Autodesk Inventor part; units mm, degrees
ref_plane "YZ Plane" through (0, 0, 0) normal (1, 0, 0) x (0, 1, 0)
ref_plane "XZ Plane" through (0, 0, 0) normal (0, 1, 0) x (-1, 0, 0)
ref_plane "XY Plane" through (0, 0, 0) normal (0, 0, 1) x (1, 0, 0)
sketch "Sketch1" plane through (0, 0, 0) normal (0, 1, 0) x (-1, 0, 0)
  line L0 (25, -25) -> (-25, -25)
  line L1 (-25, -25) -> (-25, 25)
  line L2 (-25, 25) -> (25, 25)
  line L3 (25, 25) -> (25, -25)
  line L4 (25, -25) -> (-25, 25) construction
  line L5 (-25, -25) -> (25, 25) construction
  point P0 (0, 0)
  dimension "d0" = 50
  dimension "d1" = 50
extrude "Extrusion1" add sketch "Sketch1" along normal blind 10
sketch "Sketch7" plane through (0, 0, 0) normal (0, -1, 0) x (1, 0, 0)
  circle A0 centre (0, 0) radius 11.1
  line L0 (-15.5, -15.5) -> (15.5, -15.5)
  line L1 (15.5, -15.5) -> (15.5, 15.5)
  line L2 (15.5, 15.5) -> (-15.5, 15.5)
  line L3 (-15.5, 15.5) -> (-15.5, -15.5)
  line L4 (-15.5, -15.5) -> (15.5, 15.5) construction
  line L5 (15.5, -15.5) -> (-15.5, 15.5) construction
  circle A1 centre (-15.5, 15.5) radius 1.65
  circle A2 centre (-15.5, -15.5) radius 1.65
  circle A3 centre (15.5, -15.5) radius 1.65
  circle A4 centre (15.5, 15.5) radius 1.65
  dimension "d60" = 22.2
  dimension "d61" = 31
  dimension "d62" = 31
  dimension "d63" = 3.3
  dimension "d66" = 360
extrude "Extrusion6" cut sketch "Sketch7" against normal up to next contours A0 | L3 A2 L0 | L0 A2 L3 | A3 L1 L0 | L0 L1 A3 | A1 L2 L3 | L3 L2 A1 | A4 L2 L1 | L1 L2 A4
sketch "Sketch4" plane through (0, 0, 0) normal (0, -1, 0) x (1, 0, 0)
  line L0 (25, -25) -> (25, 25)
  line L1 (0, -22.2) -> (0, 22.2) construction
  line L2 (11.5, -22.2) -> (11.5, 22.2)
  line L3 (-11.5, 22.2) -> (-11.5, -22.2)
  arc A0 (-11.5, -22.2) -> (11.5, -22.2) centre (0, -22.2) ccw
  arc A1 (11.5, 22.2) -> (-11.5, 22.2) centre (0, 22.2) ccw
  line L4 (15.5, -15.5) -> (-15.5, -15.5)
  line L5 (-15.5, -15.5) -> (-15.5, 15.5)
  line L6 (-15.5, 15.5) -> (15.5, 15.5)
  line L7 (15.5, 15.5) -> (15.5, -15.5)
  line L8 (15.5, -15.5) -> (-15.5, 15.5) construction
  line L9 (-15.5, -15.5) -> (15.5, 15.5) construction
  line L10 (-15.5, -6.7) -> (-15.5, 37.7) construction
  line L11 (-13.85, -6.7) -> (-13.85, 37.7)
  line L12 (-17.15, 37.7) -> (-17.15, -6.7)
  arc A2 (-17.15, -6.7) -> (-13.85, -6.7) centre (-15.5, -6.7) ccw
  arc A3 (-13.85, 37.7) -> (-17.15, 37.7) centre (-15.5, 37.7) ccw
  line L13 (15.5, -6.7) -> (15.5, 37.7) construction
  line L14 (17.15, -6.7) -> (17.15, 37.7)
  line L15 (13.85, 37.7) -> (13.85, -6.7)
  arc A4 (13.85, -6.7) -> (17.15, -6.7) centre (15.5, -6.7) ccw
  arc A5 (17.15, 37.7) -> (13.85, 37.7) centre (15.5, 37.7) ccw
  line L16 (-15.5, -37.7) -> (-15.5, 6.7) construction
  line L17 (-13.85, -37.7) -> (-13.85, 6.7)
  line L18 (-17.15, 6.7) -> (-17.15, -37.7)
  arc A6 (-17.15, -37.7) -> (-13.85, -37.7) centre (-15.5, -37.7) ccw
  arc A7 (-13.85, 6.7) -> (-17.15, 6.7) centre (-15.5, 6.7) ccw
  line L19 (15.5, -37.7) -> (15.5, 6.7) construction
  line L20 (17.15, -37.7) -> (17.15, 6.7)
  line L21 (13.85, 6.7) -> (13.85, -37.7)
  arc A8 (13.85, -37.7) -> (17.15, -37.7) centre (15.5, -37.7) ccw
  arc A9 (17.15, 6.7) -> (13.85, 6.7) centre (15.5, 6.7) ccw
  line L22 (25, -25) -> (-25, -25)
  line L23 (-25, -25) -> (-25, 25)
  line L24 (-25, 25) -> (25, 25)
  line L25 (25, 25) -> (25, -25)
  line L26 (25, -25) -> (-25, 25) construction
  line L27 (-25, -25) -> (25, 25) construction
  line L28 (0, 0) -> (0, 25)
  line L29 (0, 0) -> (-25, 0)
  line L30 (0, 0) -> (25, 0)
  line L31 (0, 0) -> (0, -25)
  dimension "d25" = 22.2
  dimension "d26" = 23
  dimension "d27" = 31
  dimension "d28" = 31
  dimension "d29" = 22.2
  dimension "d30" = 3.3
  dimension "d31" = 22.2
  dimension "d32" = 3.3
  dimension "d33" = 22.2
  dimension "d34" = 3.3
  dimension "d35" = 22.2
  dimension "d36" = 3.3
equation "\"d60\" = center_hole"
equation "\"d63\" = mount_hole"
equation "\"d25\" = center_hole"
equation "\"d29\" = center_hole"
equation "\"d31\" = center_hole"
equation "\"d33\" = center_hole"
equation "\"d35\" = center_hole"
equation "\"center_hole\" = 22.2"
equation "\"mount_hole\" = 3.3"
properties part number "nema17gen"
Could you check a few things on this model? Use its own coordinates, in mm. Give positions to 0.01 mm unless a question says otherwise; leave off trailing zeros. Order: outer loops, then holes, each group sorted by start corner. A loop starts at its lowest first (then second) coordinate and runs counter-clockwise, first axis right, second up. Notation, with made-up numbers: (-12.75, -17) - (41.25, -17) arc R26 ccw to (41.25, 22) - close; hole circle Ø3 at (-18, 6). An arc over 180 degrees is marked (long way). One line per item, written item: value. Start each with the question number.
1. If I drill on probe 1 along X at (y, z) = (3.25, 15.5); probe 2 along Z at (x, y) = (8.5, 9.75), over which ranges is the centre line in solid material (lowest first)?
2. Thinking about a two-plate mould opening in X: for faces 1 (the face through (-25, 5, 0)), 2 (the face through (-13.976, 4.93, 14.868)), 3 (the face through (0, 5, -25)), which applies, +X half, -X half, draft (parallel to the pull), parting line (faces both ways), or undercut?
3. Imagine slicing it at D-D on z = 0. List the corners of the cut face in (x, y) for me.
4. Imagine slicing it at A-A on x = 0. List the corners of the cut face in (y, z) for me, plus the area to 3 significant figures.
5. For P1, Ø2.5, axis at x = 15.5, z = -15.5, coming from the -Y side, with a flat end and sliding along its axis, tell me the tip position at first contact or that it passes through.
6. Imagine slicing it at C-C on y = 2.25. List the corners of the cut face in (x, z) for me, plus the area to 3 significant figures.
7. Imagine slicing it at B-B on z = 15.5. List the corners of the cut face in (x, y) for me, plus the area to 3 significant figures.
Values:
1. probe 1: -25 to -17.15, -13.85 to 13.85, 17.15 to 25
1. probe 2: -25 to -7.14, 7.14 to 25
2. face 1: -X half
2. face 2: undercut
2. face 3: draft
3. outline: (-25, 0) - (-11.1, 0) - (-11.1, 10) - (-25, 10) - close; (11.1, 0) - (25, 0) - (25, 10) - (11.1, 10) - close
4. outline: (0, -25) - (10, -25) - (10, -11.1) - (0, -11.1) - close; (0, 11.1) - (10, 11.1) - (10, 25) - (0, 25) - close
4. area: 278 mm²
5. P1: through
6. outline: (-25, -25) - (25, -25) - (25, 25) - (-25, 25) - close; hole circle Ø3.3 at (-15.5, -15.5); hole circle Ø3.3 at (-15.5, 15.5); hole circle Ø22.2 at (0, 0); hole circle Ø3.3 at (15.5, -15.5); hole circle Ø3.3 at (15.5, 15.5)
6. area: 2,080 mm²
7. outline: (-25, 0) - (-17.15, 0) - (-17.15, 10) - (-25, 10) - close; (-13.85, 0) - (13.85, 0) - (13.85, 10) - (-13.85, 10) - close; (17.15, 0) - (25, 0) - (25, 10) - (17.15, 10) - close
7. area: 434 mm²
